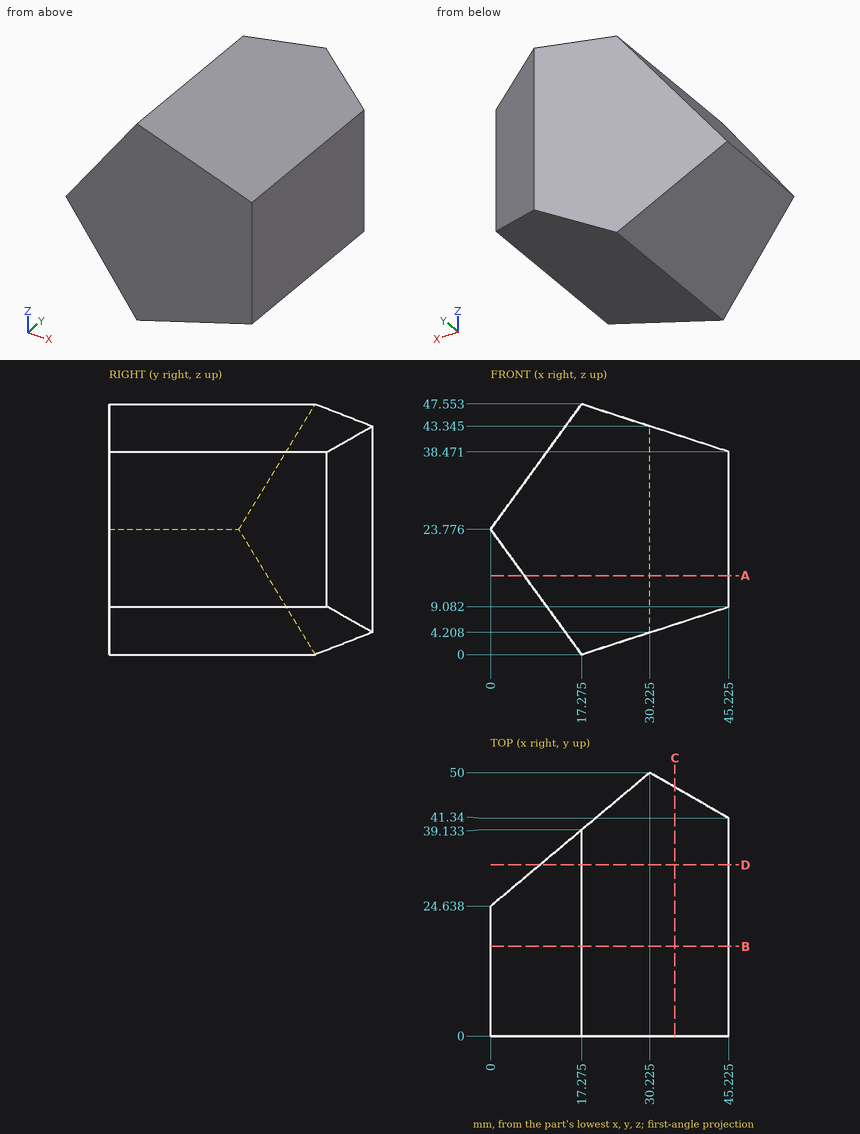
Check sheet for the drawn part. Datum: minimum x, y, z corner. Units: mm. Give positions to 0.01 mm unless a question says otherwise; leave off trailing zeros. Loops run counter-clockwise (first coordinate to the right, second up) from the corner with the lowest first, then second, coordinate; pieces in that order, holes last.
1) Sectioned sample at D-D, the plane y = 32.5. Enter the section's corners in (x, z) (1 decimal), then the cut area to 3 significant figures.
2) Depth check by flat-ended pin: pin 1 Ø6 at (x, y) = (35, 45) entering from +Z; pin 2 Ø3 at (x, z) = (12.5, 29.5) entering from +Y (1 decimal); pin 3 Ø1 at (x, y) = (7, 25.5) entering from -Z (1 decimal). Enter the tip coordinate at first touch or a pass-through.
3) Sectioned sample at B-B, the plane y = 17. Enter the section's corners in (x, z) (1 decimal).
4) Sectioned sample at A-A, the plane z = 15. Enter the section's corners in (x, y) (1 decimal), then the cut area to 3 significant figures.
5) Thickness scan on line 1 along Z through (x, y) = (25, 31.5); line 2 along Y through (x, z) = (23.5, 9.5) (1 decimal); line 3 along Z through (x, y) = (17, 24.5) (1 decimal). Record the ranges inside material, lowest first.
6) Sectioned sample at C-C, the plane x = 35. Enter the section's corners in (y, z).
Answers:
1. outline: (9.4, 10.9) - (17.3, 0) - (45.2, 9.1) - (45.2, 38.5) - (17.3, 47.6) - (9.4, 36.7) - close
1. area: 1,370 mm2
2. pin 1: stops at z = 42.77
2. pin 2: stops at y = 36.4
2. pin 3: stops at z = 13.5
3. outline: (0, 23.8) - (17.3, 0) - (45.2, 9.1) - (45.2, 38.5) - (17.3, 47.6) - close
4. outline: (6.4, 0) - (45.2, 0) - (45.2, 41.3) - (30.2, 50) - (6.4, 30) - close
4. area: 1,640 mm2
5. line 1: z = 2.51 to 45.04
5. line 2: y = 0 to 44.4
5. line 3: z = 0.4 to 47.2
6. outline: (0, 5.76) - (47.24, 5.76) - (47.24, 41.79) - (0, 41.79) - close
